The listing builds one solid part. Answer for the finished solid, in the listing's coordinates (mm). Face numbers are marked on the shaded views. A direction names the side the tool comes from. Coordinates: 2 decimals unless noted, no trailing zeros. Loops run counter-clockwise (first coordinate to the right, second up) from the corner with the lowest first, then second, coordinate; pieces in that order, holes last. Notation, with made-up numbers: (51.25, 47) -> (97.25, 47) arc R30 ccw to (97.25, 72) -> close; hole circle Ø5 at (-9.5, 8.25). An arc over 180 degrees is marked (long way). Answer in a Markdown table with one row per item.
```python
from build123d import *

# Parameters (mm, degrees)
F2_R    = 6
F3_SIZE = 10
F4_T    = -2.5


with BuildPart() as f1:
    # F0 (on Top) → F1 (revolve)
    with BuildSketch(Plane.XY):
        Polygon((-120.2378347516, 63.5438784957), (-120.2378347516, 6.4126844518), (-32.5006470084, -37.3101644218), (-32.5006470084, 0), (0, 0), (0, 63.5438784957), align=None)
    revolve(axis=Axis((0, 18.9465675503, 0), (0, -1, 0)))

    # F2
    f2_edges = [f1.edges().sort_by_distance(p)[0] for p in [
        (120.237835, 6.412684, 0),
    ]]
    fillet(f2_edges, radius=F2_R)

    # F3
    f3_edges = [f1.edges().sort_by_distance(p)[0] for p in [
        (32.500647, -37.310164, 0),
    ]]
    chamfer(f3_edges, length=F3_SIZE)

    # F4
    f4_openings = [f1.faces().sort_by_distance(p)[0] for p in [
        (0, 63.543878, 0),
    ]]
    offset(amount=F4_T, openings=f4_openings, kind=Kind.INTERSECTION)


solid = f1.part
```
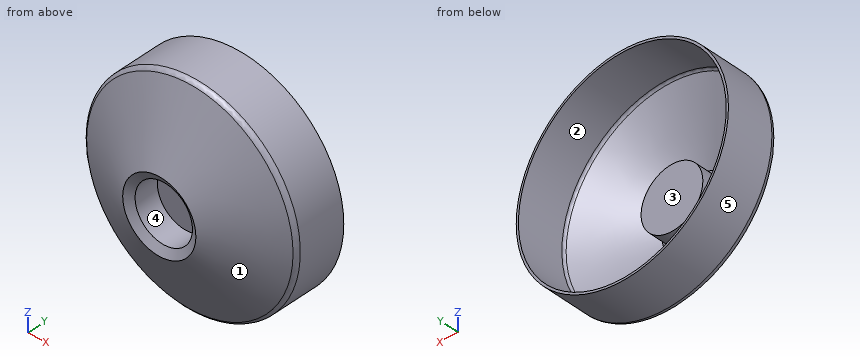
Item 1: A cutting plane is placed at A-A, the plane y = -4. Determine the outline of the cut face in (x, z), plus the area to 3 significant figures.
Findings below:
| item | result |
|---|---|
| outline | circle Ø198.69 at (0, 0); circle Ø70 at (0, 0); hole circle Ø187.48 at (0, 0); hole circle Ø65 at (0, 0) |
| area | 3,930 mm2 |
Item 2: Find the intervals of material crossed by probe 1 along X at (y, z) = (35.5, 0); probe 2 along X at (y, z) = (-10, 0), in increasing order.
Findings below:
| item | result |
|---|---|
| probe 1 | x = -120.24 to -117.74, 117.74 to 120.24 |
| probe 2 | x = -87.3 to -81.7, -35 to -32.5, 32.5 to 35, 81.7 to 87.3 |
Item 3: Determine the mould class of the marked faces 1 and 2 for opening direction X: +X half, -X half, draft (parallel to the pull), parting line (faces both ways), or undercut.
Findings below:
| item | result |
|---|---|
| face 1 | parting line |
| face 2 | undercut |
Item 4: Flat-ended cylindrical pins translate along their axes: pin 1 Ø3 at (x, y) = (-75.5, 40.5) entering from +Z; pin 2 Ø4 at (y, z) = (31, 59.5) entering from +X; pin 3 Ø6 at (x, z) = (-39.5, -84) entering from -Y. Find the tip coordinate at first contact, or state that the pin passes through.
Findings below:
| item | result |
|---|---|
| pin 1 | stops at z = 94.77 |
| pin 2 | stops at x = 105.6 |
| pin 3 | stops at y = -8.74 |
Item 5: A tool of negligible diameter and unlimited length cuts with its end or side. For the marked faces 3, 4 and 5, from which of +Z, -Z, +X, -X, +Y, -Y can it reach the whole face along a straight path? Write none if from no direction.
Findings below:
| item | result |
|---|---|
| face 3 | +Y |
| face 4 | -Y |
| face 5 | +Y, -Y |
Item 6: A cutting plane is placed at B-B, the plane y = 54.5. Determine the outline of the cut face in (x, z).
Findings below:
| item | result |
|---|---|
| outline | circle Ø240.48 at (0, 0); hole circle Ø235.48 at (0, 0) |
Item 7: A cutting plane is placed at C-C, the plane y = -20.5. Determine the outline of the cut face in (x, z), plus the area to 3 significant figures.
Findings below:
| item | result |
|---|---|
| outline | circle Ø132.47 at (0, 0); circle Ø70 at (0, 0); hole circle Ø121.26 at (0, 0); hole circle Ø65 at (0, 0) |
| area | 2,760 mm2 |
